The listing builds one solid part. Answer for the finished solid, in the listing's coordinates (mm). Face numbers are marked on the shaded views. A direction names the side the tool comes from. Give positions to 0.01 mm unless a question says otherwise; leave off trailing zeros. Loops run counter-clockwise (first coordinate to the right, second up) from the corner with the lowest first, then second, coordinate; pieces in that order, holes last. Notation, with made-up numbers: M 25,-7 L 38,-7 A34 cw 38,32 Z; hole C 15.5,82 d3. An arc over 180 degrees is marked long. Use one line per item in the form item = value. Start each with the question number.
1. Straight lines are drawn through the part: line 1 (Z direction, x = 2.75, y = -1.75); line 2 (Z direction, x = -8.25, y = -5); line 3 (X direction, y = -5.75, z = 16.25). For each, find the intervals that lie inside material, in ascending order. Write a range as from..to.
2. For the marked faces 1, 2 and 3, determine the directions among +Z, -Z, +X, -X, +Y, -Y from which every point of the face is accessible in a straight line to the end or side of a thin tool.
3. The part is cut by section D-D (z = 20). Write down the section's boundary in (x, y), and give its area (3 significant figures).
4. Each of these flat-tipped pins is pushed along its axis until it touches: pin 1 Ø0.5 at (x, z) = (-10.5, 24.5) entering from +Y; pin 2 Ø3 at (y, z) = (-3.5, 20) entering from -X; pin 3 Ø1 at (y, z) = (-2, 19) entering from +X. Where does it stop, or does it pass through?
5. The part is cut by section C-C (x = -7.75). Write down the section's boundary in (y, z).
6. The part is cut by section B-B (z = 23.75). Write down the section's boundary in (x, y).
7. The part is cut by section A-A (x = 2). Write down the section's boundary in (y, z), and give its area (4 significant figures).
from build123d import *

# Parameters (mm, degrees)
F0_W      = 22
F0_H      = 22
F1_DEPTH  = 11.5
F3_DEPTH  = 4
F4_R      = 2
F5_DEPTH  = 3
F6_W      = 11.5
F6_H      = 2.5
F7_DEPTH  = 4
F8_W      = 11.5
F8_H      = 3
F9_DEPTH  = 4
F11_DEPTH = 25.4
F13_DEPTH = 25.4


with BuildPart() as f1:
    # F0 (on Front) → F1 (new body)
    with BuildSketch(Plane.XZ):
        with Locations((-11, 11)):
            Rectangle(F0_W, F0_H)
    extrude(amount=F1_DEPTH)

    # F2 (on face) → F3 (join)
    with BuildSketch(Plane.XY.offset(22)):
        with BuildLine():
            ThreePointArc((-10.8406771994, -7.6998017434), (-11.9992952148, -5.6490453843), (-10.9393399136, -3.5455977121))
            ThreePointArc((-10.9393399136, -3.5455977121), (-11.0408940925, -3.3153099489), (-11.1524285962, -3.0896869013))
            ThreePointArc((-11.1524285962, -3.0896869013), (-13.2695889812, -0.8327192312), (-16.25, 0))
            ThreePointArc((-16.25, 0), (-20.3158639918, -1.6841360082), (-22, -5.75))
            ThreePointArc((-22, -5.75), (-20.3158639918, -9.8158639918), (-16.25, -11.5))
            ThreePointArc((-16.25, -11.5), (-13.1187622002, -10.5726393024), (-10.9975372249, -8.0896869013))
            ThreePointArc((-10.9975372249, -8.0896869013), (-10.9155440273, -7.8961778759), (-10.8406771994, -7.6998017434))
        make_face()
        with BuildLine():
            ThreePointArc((-10.8406771994, -7.6998017434), (-10.5858095855, -6.7396701209), (-10.5, -5.75))
            ThreePointArc((-10.5, -5.75), (-10.6109045275, -4.6261217808), (-10.9393399136, -3.5455977121))
            ThreePointArc((-10.9393399136, -3.5455977121), (-11.9992952148, -5.6490453843), (-10.8406771994, -7.6998017434))
        make_face()
        with BuildLine():
            ThreePointArc((-10.9393399136, -3.5455977121), (-10.6109045275, -4.6261217808), (-10.5, -5.75))
            ThreePointArc((-10.5, -5.75), (-10.5858095855, -6.7396701209), (-10.8406771994, -7.6998017434))
            ThreePointArc((-10.8406771994, -7.6998017434), (-10.1981091944, -7.9902375782), (-9.5, -8.0896869013))
            ThreePointArc((-9.5, -8.0896869013), (-7.732233047, -7.3574538542), (-7, -5.5896869013))
            ThreePointArc((-7, -5.5896869013), (-7.732233047, -3.8219199483), (-9.5, -3.0896869013))
            ThreePointArc((-9.5, -3.0896869013), (-10.2549096062, -3.2063884545), (-10.9393399136, -3.5455977121))
        make_face()
        with BuildLine():
            ThreePointArc((-11.1524285962, -3.0896869013), (-11.0408940925, -3.3153099489), (-10.9393399136, -3.5455977121))
            ThreePointArc((-10.9393399136, -3.5455977121), (-10.2549096062, -3.2063884545), (-9.5, -3.0896869013))
            Line((-9.5, -3.0896869013), (-11.1524285962, -3.0896869013))
        make_face()
        with BuildLine():
            ThreePointArc((-9.5, -8.0896869013), (-10.1981091944, -7.9902375782), (-10.8406771994, -7.6998017434))
            ThreePointArc((-10.8406771994, -7.6998017434), (-10.9155440273, -7.8961778759), (-10.9975372249, -8.0896869013))
            Line((-10.9975372249, -8.0896869013), (-9.5, -8.0896869013))
        make_face()
    extrude(amount=F3_DEPTH)

    # F4 (on face) → F5 (join)
    with BuildSketch(Plane.XY.offset(26)):
        with Locations((-16.25, -5.75)):
            Circle(F4_R)
    extrude(amount=F5_DEPTH)

    # F6 (on face) → F7 (join)
    with BuildSketch(Plane.YZ):
        with Locations((-5.75, 16.75)):
            Rectangle(F6_W, F6_H)
    extrude(amount=F7_DEPTH)

    # F8 (on face) → F9 (join)
    with BuildSketch(Plane(origin=(-22, 0, 0), x_dir=(0, -1, 0), z_dir=(-1, 0, 0))):
        with Locations((5.75, 16.5)):
            Rectangle(F8_W, F8_H)
    extrude(amount=F9_DEPTH)

    # F10 (on face) → F11 (cut)
    with BuildSketch(Plane.XY.offset(18)):
        with BuildLine():
            ThreePointArc((-24.8660254038, -6.25), (-23.7411809549, -6.7159258263), (-23, -5.75))
            ThreePointArc((-23, -5.75), (-23.7411809549, -4.7840741737), (-24.8660254038, -5.25))
            ThreePointArc((-24.8660254038, -5.25), (-25, -5.75), (-24.8660254038, -6.25))
        make_face()
        with BuildLine():
            ThreePointArc((-24.8660254038, -6.25), (-25, -5.75), (-24.8660254038, -5.25))
            Line((-24.8660254038, -5.25), (-26, -5.25))
            Line((-26, -5.25), (-26, -6.25))
            Line((-26, -6.25), (-24.8660254038, -6.25))
        make_face()
    extrude(amount=-F11_DEPTH, mode=Mode.SUBTRACT)

    # F12 (on face) → F13 (cut)
    with BuildSketch(Plane.XY.offset(18)):
        with BuildLine():
            ThreePointArc((2.8660254038, -6.25), (2.9659258263, -6.0088190451), (3, -5.75))
            ThreePointArc((3, -5.75), (2.9659258263, -5.4911809549), (2.8660254038, -5.25))
            ThreePointArc((2.8660254038, -5.25), (1, -5.75), (2.8660254038, -6.25))
        make_face()
        with BuildLine():
            ThreePointArc((2.8660254038, -5.25), (2.9659258263, -5.4911809549), (3, -5.75))
            ThreePointArc((3, -5.75), (2.9659258263, -6.0088190451), (2.8660254038, -6.25))
            Line((2.8660254038, -6.25), (4, -6.25))
            Line((4, -6.25), (4, -5.25))
            Line((4, -5.25), (2.8660254038, -5.25))
        make_face()
    extrude(amount=-F13_DEPTH, mode=Mode.SUBTRACT)


solid = f1.part
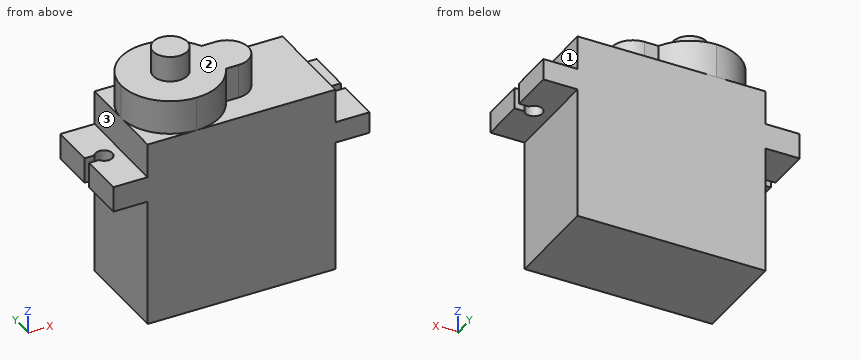
Derived:
q1.line_1 = 15.5..18
q1.line_2 = 0..26
q1.line_3 = -23..1
q2.face_1 = +Z, +X, +Y, -Y
q2.face_2 = +Z
q2.face_3 = +Z, -X, +Y, -Y
q3.outline = M -22,-11.5 L 0,-11.5 L 0,0 L -22,0 Z
q3.area = 253 mm2
q4.pin_1 = -3.09
q4.pin_2 = -22
q4.pin_3 = 0
q5.outline = M -11.5,0 L 0,0 L 0,22 L -3.8,22 L -3.8,26 L -7.38,26 L -7.38,22 L -11.5,22 Z
q6.outline = M -11.15,-3.09 A5.75 ccw long -11,-8.09 L -9.5,-8.09 A2.5 ccw -9.5,-3.09 Z
q7.outline = M -11.5,15.5 L -6.75,15.5 L -6.75,18 L -11.5,18 Z; M -4.75,15.5 L 0,15.5 L 0,18 L -4.75,18 Z
q7.area = 23.75 mm2
